Part model, mm, in its own coordinate system. A direction names the side the tool comes from. Give positions to 0.01 mm unless a question says otherwise; leave off trailing zeros. Loops run counter-clockwise (first coordinate to the right, second up) from the corner with the lowest first, then second, coordinate; pieces in that order, holes last. Notation, with made-up numbers: (-21.5, -23) -> (4.5, -23) arc R10 cw to (4.5, -5) -> close; hole circle Ø7 at (65.25, 60). An arc over 180 degrees is marked (long way). One line per question, with ' | ' between items.
Autodesk Inventor part; units mm, degrees
ref_plane "YZ Plane" through (0, 0, 0) normal (1, 0, 0) x (0, 1, 0)
ref_plane "XZ Plane" through (0, 0, 0) normal (0, 1, 0) x (-1, 0, 0)
ref_plane "XY Plane" through (0, 0, 0) normal (0, 0, 1) x (1, 0, 0)
sketch "Esquisse2" plane through (0, 0, 0) normal (0, 0, 1) x (1, 0, 0)
  line L0 (0, 0) -> (0, 50)
  line L1 (0, 50) -> (290, 0)
  line L2 (290, 0) -> (0, 0)
  dimension "d0" = 290
  dimension "d1" = 50
extrude "Extrusion1" add sketch "Esquisse2" along normal blind 40
sketch "Esquisse3" plane through (0, 50, 40) normal (0.1699069, 0.9854601, 0) x (0.9854601, -0.1699069, 0)
  line L0 (0, 40) -> (0, 0)
  line L1 (0, 2) -> (294.2788, 2)
  line L2 (294.2788, 40) -> (294.2788, 0)
  line L3 (0, 38) -> (294.2788, 38)
  line L4 (0, 40) -> (294.2788, 40)
  line L5 (294.2788, 0) -> (0, 0)
  point P0 (8.4953, 40)
  dimension "d5" = 2
  dimension "d6" = 2
extrude "Extrusion2" add sketch "Esquisse3" along normal blind 5 contours L4 L2 L3 L0 | L1 L2 L5 L0
properties part number "rampe-rendmonnaie"
1) Pin check, flat tips, straight feed: P1, Ø1, axis at x = 45.5, z = 19.5, coming from the -Y side; P2, Ø5, axis at x = 233.5, z = 9, coming from the +Y side; P3, Ø10, axis at x = 89, z = 24.5, coming from the +Y side. Stop position of each tip, or through.
Found:
P1: y = 0 | P2: y = 10.17 | P3: y = 35.52
2) Drill centre lines: line 1 (Z direction, x = 142.5, y = 28); line 2 (Y direction, x = 41, z = 35); line 3 (Y direction, x = 269.5, z = 3). Where is each one in solid material? Low to high.
Found:
line 1: 0 to 2, 38 to 40 | line 2: 0 to 42.93 | line 3: 0 to 3.53
3) Tool access for faces 4 (the flat face through (142.97, 25.35, 19.75)), 5 (the flat face through (143.82, 30.277, 38.986)): list every direction of +Z, -Z, +X, -X, +Y, -Y with a clear straight run to the whole face (end or side of a thin tool).
Found:
face 4: +X, +Y | face 5: +Z, -Z, +X, +Y
4) Saw through at A-A (y = 37). Give the cut face in (x, z).
Found:
outline: (0, 0) -> (104.83, 0) -> (104.83, 2) -> (75.4, 2) -> (75.4, 38) -> (104.83, 38) -> (104.83, 40) -> (0, 40) -> close
5) Pull direction Z, two halves, no side cores. Call faces 1 (the flat face through (143, 28, 2)), 2 (the flat face through (111, 22, 40)), 3 (the flat face through (147, 0, 20)): pulls with the +Z half, pulls with the -Z half, needs draft (parallel to the pull), parting line crosses it, or undercut.
Found:
face 1: undercut | face 2: pulls with the +Z half | face 3: needs draft
6) Saw through at C-C (z = 20). Give the cut face in (x, y).
Found:
outline: (0, 0) -> (290, 0) -> (0, 50) -> close
7) Saw through at B-B (x = 104). Give the cut face in (y, z), and give its area (3 significant figures).
Found:
outline: (0, 0) -> (37.14, 0) -> (37.14, 2) -> (32.07, 2) -> (32.07, 38) -> (37.14, 38) -> (37.14, 40) -> (0, 40) -> close | area: 1,300 mm2
